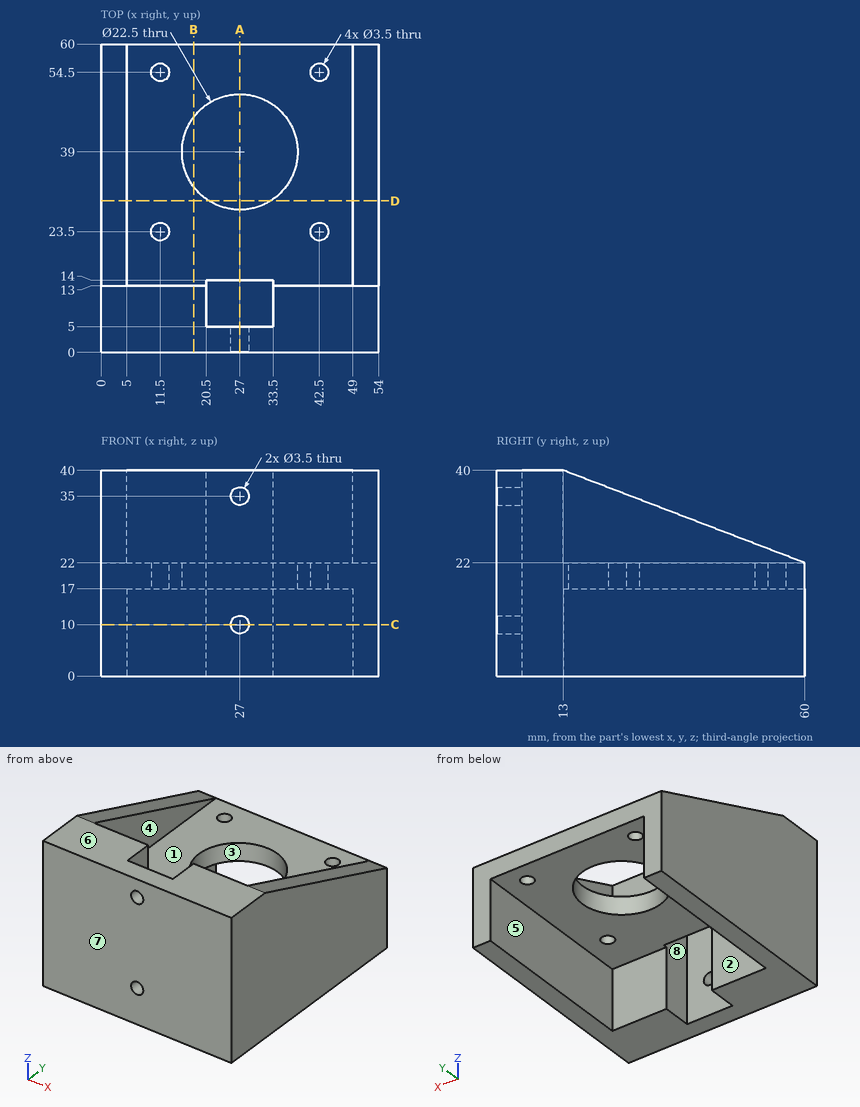
Here's the drawing with two shaded views (mm, measured from the low corner). I have some questions. A direction names the side the tool comes from. Round coordinates to 2 decimals unless told otherwise and drop trailing zeros. Loops run counter-clockwise (first coordinate to the right, second up) from the corner with the lowest first, then second, coordinate; pieces in that order, holes last. Notation, with made-up numbers: M 12,-32 L 24,-32 A7 cw 24,-19 Z; hole C 41,72.25 d7. An arc over 180 degrees is marked long. Answer as a JSON object with one key per item and string values. Group by question number.
Q1. Imagine slicing it at D-D, the plane y = 29.5. Please give me the cut outline in (x, z).
Q2. We'd pull the mould along Y, two halves only. Please class the marked faces 1, 2 and 3: +Y half, -Y half, draft (parallel to the pull), parting line (faces both ways), or undercut.
Q3. Will these pins go through, and if not, where does the flat tip stop? pin 1 (3 mm diameter, centred on x = 16.5, z = 27, fed in from -Y); pin 2 (17 mm diameter, centred on x = 37.5, z = 34, fed in from +Y); pin 3 (5 mm diameter, centred on x = 36.5, y = 54, fed in from +Z); pin 4 (5.5 mm diameter, centred on x = 27, z = 10, fed in from +Y).
Q4. Imagine slicing it at C-C, the plane z = 10. Please give me the cut outline in (x, y).
Q5. Imagine slicing it at B-B, the plane x = 18. Please give me the cut outline in (y, z).
Q6. Please list where these lines run through material, in increasing order: L1, parallel to X at y = 23.5, z = 18.5; L2, parallel to Z at x = 27, y = 1.5; L3, parallel to X at y = 39, z = 19.55.
Q7. On a 3-axis mill with a long thin cutter (end or side, diameter ignored), from which of +Z, -Z, +X, -X, +Y, -Y can I reach the whole of each face in a straight line? I mean the marked faces 4, 5, 6, 7 and 8. Say none if no direction works.
Q8. Imagine slicing it at A-A, the plane x = 27. Please give me the cut outline in (y, z), then the cut area to 4 significant figures.
Findings:
{
 "1": {"outline": "M 0,0 L 5,0 L 5,17 L 20.97,17 L 20.97,22 L 5,22 L 5,33.68 L 0,33.68 Z; M 33.03,17 L 49,17 L 49,0 L 54,0 L 54,33.68 L 49,33.68 L 49,22 L 33.03,22 Z"},
 "2": {"face 1": "draft", "face 2": "+Y half", "face 3": "undercut"},
 "3": {"pin 1": "stops at y = 0", "pin 2": "stops at y = 13", "pin 3": "stops at z = 22", "pin 4": "stops at y = 5"},
 "4": {"outline": "M 0,0 L 25.25,0 L 25.25,5 L 20.5,5 L 20.5,13 L 5,13 L 5,60 L 0,60 Z; M 28.75,0 L 54,0 L 54,60 L 49,60 L 49,13 L 33.5,13 L 33.5,5 L 28.75,5 Z"},
 "5": {"outline": "M 0,0 L 13,0 L 13,17 L 32.25,17 L 32.25,22 L 13,22 L 13,40 L 0,40 Z; M 45.75,17 L 60,17 L 60,22 L 45.75,22 Z"},
 "6": {"L1": "x = 0 to 9.75, 13.25 to 40.75, 44.25 to 54", "L2": "z = 0 to 8.25, 11.75 to 33.25, 36.75 to 40", "L3": "x = 0 to 15.75, 38.25 to 54"},
 "7": {"face 4": "+Z, +Y", "face 5": "-Z, +Y", "face 6": "+Z, +X, -X, +Y, -Y", "face 7": "+Z, -Z, +X, -X, -Y", "face 8": "+Z, -Z"},
 "8": {"outline": "M 0,0 L 5,0 L 5,8.25 L 0,8.25 Z; M 0,11.75 L 5,11.75 L 5,33.25 L 0,33.25 Z; M 0,36.75 L 5,36.75 L 5,40 L 0,40 Z; M 14,17 L 27.75,17 L 27.75,22 L 14,22 Z; M 50.25,17 L 60,17 L 60,22 L 50.25,22 Z", "area": "282.5 mm2"}
}
